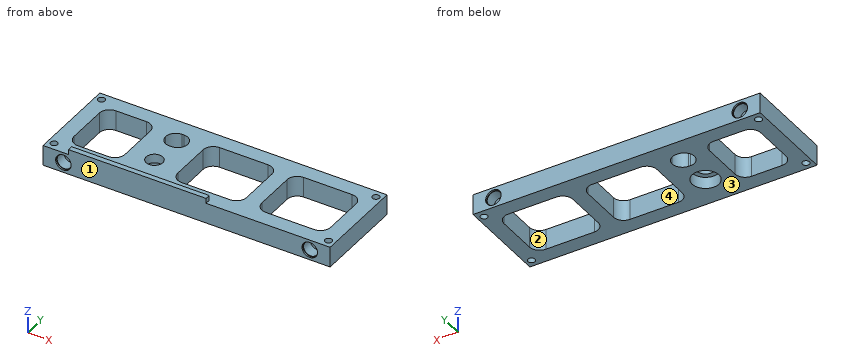
from build123d import *

# Parameters (mm, degrees)
F0_W      = 112.7
F0_H      = 36
F1_DEPTH  = 8
F3_W      = 54
F3_H      = 2
F4_DEPTH  = 2
F5_R      = 3.27
F6_DEPTH  = 8.001
F7_R      = 1.375
F8_DEPTH  = 10.001
F10_R     = 5.25
F11_DEPTH = 4.5
F9_W      = 20
F9_H      = 24
F9_W_2    = 27
F9_W_3    = 8.7
F9_H_2    = 8
F12_DEPTH = 10.001
F13_R     = 3.99999
F14_R     = 2.795
F15_DEPTH = 4.8
F16_R     = 2.795
F17_DEPTH = 4.8
F18_R     = 3.05
F19_DEPTH = 0.6
F20_R     = 3.05
F21_DEPTH = 0.6


# Not quite as in the source:
# - a fillet or chamfer is up to 0.001 mm smaller than in the source, because OpenCascade refuses the exact size


with BuildPart() as f1:
    # F0 (on Top) → F1 (new body)
    with BuildSketch(Plane.XY):
        Rectangle(F0_W, F0_H)
    extrude(amount=F1_DEPTH)

    # F3 (on face) → F4 (join)
    with BuildSketch(Plane.XY.offset(8)):
        with Locations((-19.35, -17)):
            Rectangle(F3_W, F3_H)
    extrude(amount=F4_DEPTH)

    # F5 (on face) → F6 (cut, through all)
    with BuildSketch(Plane.XY.offset(8)):
        with Locations((-20.35, -5.5)):
            Circle(F5_R)
    extrude(amount=-F6_DEPTH, mode=Mode.SUBTRACT)

    # F7 (on face) → F8 (cut, through all)
    with BuildSketch(Plane(origin=(0, 0, 0), x_dir=(1, 0, 0), z_dir=(0, 0, -1))):
        with Locations((-53.85, 15)):
            Circle(F7_R)
        with Locations((-53.85, -15)):
            Circle(F7_R)
        with Locations((53.85, 15)):
            Circle(F7_R)
        with Locations((53.85, -15)):
            Circle(F7_R)
    extrude(amount=-F8_DEPTH, mode=Mode.SUBTRACT)

    # F10 (on face) → F11 (cut)
    with BuildSketch(Plane(origin=(0, 0, 0), x_dir=(1, 0, 0), z_dir=(0, 0, -1))):
        with Locations((-20.35, 5.5)):
            Circle(F10_R)
    extrude(amount=-F11_DEPTH, mode=Mode.SUBTRACT)

    # F9 (on face) → F12 (cut, through all)
    with BuildSketch(Plane(origin=(0, 0, 0), x_dir=(1, 0, 0), z_dir=(0, 0, -1))):
        with Locations((-40.35, 0)):
            Rectangle(F9_W, F9_H)
        with Locations((3.85, 0)):
            Rectangle(F9_W_2, F9_H)
        with Locations((36.85, 0)):
            Rectangle(F9_W_2, F9_H)
        with Locations((-20, -8)):
            Rectangle(F9_W_3, F9_H_2)
    extrude(amount=-F12_DEPTH, mode=Mode.SUBTRACT)

    # F13 (radius 4 in the source; OpenCascade refuses exactly that, so slightly less here)
    f13_edges = [f1.edges().sort_by_distance(p)[0] for p in [
        (-30.35, -12, 4),
        (-50.35, -12, 4),
        (-50.35, 12, 4),
        (-30.35, 12, 4),
        (-24.35, 4, 4),
        (-9.65, -12, 4),
        (23.35, -12, 4),
        (-9.65, 12, 4),
        (-24.35, 12, 4),
        (17.35, -12, 4),
        (50.35, -12, 4),
        (50.35, 12, 4),
        (23.35, 12, 4),
        (-15.65, 4, 4),
        (-15.65, 12, 4),
        (17.35, 12, 4),
    ]]
    fillet(f13_edges, radius=F13_R)

    # F14 (on face) → F15 (cut)
    with BuildSketch(Plane.XZ.offset(18)):
        with Locations((48.35, 4)):
            Circle(F14_R)
        with Locations((-48.35, 4)):
            Circle(F14_R)
    extrude(amount=-F15_DEPTH, mode=Mode.SUBTRACT)

    # F16 (on face) → F17 (cut)
    with BuildSketch(Plane(origin=(0, 18, 0), x_dir=(-1, 0, 0), z_dir=(0, 1, 0))):
        with Locations((48.35, 4)):
            Circle(F16_R)
        with Locations((-48.35, 4)):
            Circle(F16_R)
    extrude(amount=-F17_DEPTH, mode=Mode.SUBTRACT)

    # F18 (on face) → F19 (cut)
    with BuildSketch(Plane.XZ.offset(18)):
        with Locations((-48.35, 4)):
            Circle(F18_R)
        with Locations((48.35, 4)):
            Circle(F18_R)
    extrude(amount=-F19_DEPTH, mode=Mode.SUBTRACT)

    # F20 (on face) → F21 (cut)
    with BuildSketch(Plane(origin=(0, 18, 0), x_dir=(-1, 0, 0), z_dir=(0, 1, 0))):
        with Locations((-48.35, 4)):
            Circle(F20_R)
        with Locations((48.35, 4)):
            Circle(F20_R)
    extrude(amount=-F21_DEPTH, mode=Mode.SUBTRACT)


solid = f1.part
Here's how the part is built. I have some questions about the finished solid (model axes, mm). Face numbers are marked on the shaded views. A direction names the side the tool comes from. Round coordinates to 2 decimals unless told otherwise and drop trailing zeros. Write each loop counter-clockwise with the first axis right and the second up, starting at its lowest first coordinate (ties: lowest second). Pieces come first, ordered by that corner, then holes.
1. Suppose I cut it at D-D (x = -37). List the corners of the cut face in (y, z) for me, and give its area (3 significant figures).
2. If we mould it in two halves opening along X, with no side actions, what happens to the marked faces 1 and 2? For each: released by +X, released by -X, zero draft, split by the parting line, or undercut.
3. Will these pins go through, and if not, where does the flat tip stop? pin 1 Ø1 at (x, y) = (-13, -12.5) entering from +Z; pin 2 Ø3 at (x, z) = (48.5, 3) entering from +Y; pin 3 Ø1 at (y, z) = (-16.5, 9) entering from -X.
4. For the marked faces 3 and 4, which set-ups out of +Z, -Z, +X, -X, +Y, -Y let a thin tool reach every point of the face, with its end or its side?
5. Suppose I cut it at A-A (y = 15). List the corners of the cut face in (x, z) for me (3 decimals), and give its area (3 significant figures).
6. Suppose I cut it at B-B (x = -53.85). List the corners of the cut face in (y, z) for me (3 decimals), and give its area (3 significant figures).
7. I need wall thicknesses on L1, parallel to X at y = -5.5, z = 0.75; L2, parallel to X at y = 2, z = 5.25; L3, parallel to Z at x = 48.35, y = 17.6. Which ranges of each line are inside material? Lowest first, please.
8. Suppose I cut it at C-C (y = -5.5). List the corners of the cut face in (x, z) for me, and give its area (3 significant figures).
Answer sheet:
1. outline: (-18, 0) - (-12, 0) - (-12, 8) - (-16, 8) - (-16, 10) - (-18, 10) - close; (12, 0) - (18, 0) - (18, 8) - (12, 8) - close
1. area: 100 mm2
2. face 1: zero draft
2. face 2: undercut
3. pin 1: stops at z = 8
3. pin 2: stops at y = 13.2
3. pin 3: stops at x = -46.35
4. face 3: -Z, +X, -X, +Y, -Y
4. face 4: +Z, -Z
5. outline: (-56.35, 0) - (-55.225, 0) - (-55.225, 8) - (-56.35, 8) - close; (-52.475, 0) - (52.475, 0) - (52.475, 8) - (-52.475, 8) - close; (55.225, 0) - (56.35, 0) - (56.35, 8) - (55.225, 8) - close; hole circle Ø5.59 at (-48.35, 4); hole circle Ø5.59 at (48.35, 4)
5. area: 809 mm2
6. outline: (-18, 0) - (-16.375, 0) - (-16.375, 8) - (-18, 8) - close; (-13.625, 0) - (13.625, 0) - (13.625, 8) - (-13.625, 8) - close; (16.375, 0) - (18, 0) - (18, 8) - (16.375, 8) - close
6. area: 244 mm2
7. L1: x = -56.35 to -50.35, -30.35 to -25.6, -15.1 to -9.65, 17.35 to 23.35, 50.35 to 56.35
7. L2: x = -56.35 to -50.35, -30.35 to -9.65, 17.35 to 23.35, 50.35 to 56.35
7. L3: z = 0 to 0.95, 7.05 to 8
8. outline: (-56.35, 0) - (-50.35, 0) - (-50.35, 8) - (-56.35, 8) - close; (-30.35, 0) - (-25.6, 0) - (-25.6, 4.5) - (-23.62, 4.5) - (-23.62, 8) - (-30.35, 8) - close; (-17.08, 4.5) - (-15.1, 4.5) - (-15.1, 0) - (-9.65, 0) - (-9.65, 8) - (-17.08, 8) - close; (17.35, 0) - (23.35, 0) - (23.35, 8) - (17.35, 8) - close; (50.35, 0) - (56.35, 0) - (56.35, 8) - (50.35, 8) - close
8. area: 239 mm2
